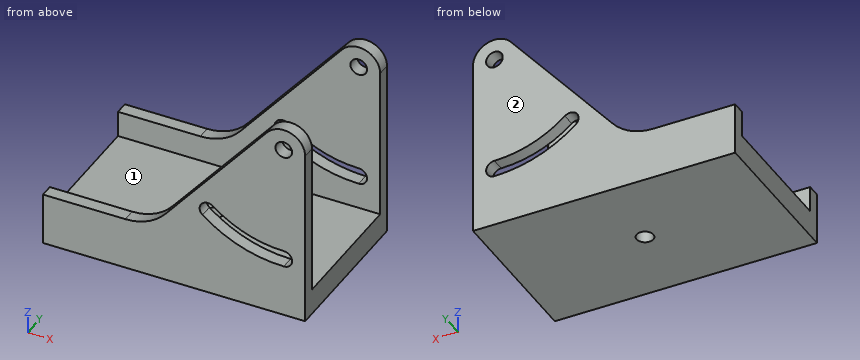
```python
from build123d import *

# Parameters (mm, degrees)
SKETCH002_W  = 100
SKETCH002_H  = 60
SKETCH002_R  = 3.175
PAD002_DEPTH = 10
SKETCH003_R  = 3.175
PAD003_DEPTH = 60
SKETCH004_W  = 50
SKETCH004_H  = 66.35
POCKET_DEPTH = 100.001


with BuildPart() as part:
    # Sketch002 → Pad002 (new body)
    with BuildSketch(Plane.XY):
        Rectangle(SKETCH002_W, SKETCH002_H)
        Circle(SKETCH002_R, mode=Mode.SUBTRACT)
    extrude(amount=PAD002_DEPTH)

    # Sketch003 (on Face1 of Pad002) → Pad003 (join)
    with BuildSketch(Plane.XZ.offset(30)):
        with BuildLine():
            ThreePointArc((50, 68.175), (44.621015, 75.856987), (35.562587, 73.429789))
            Line((-3.275594, 27.144248), (35.562587, 73.429789))
            ThreePointArc((-18.596482, 20), (-10.144117, 21.873844), (-3.275594, 27.144248))
            Line((-50, 20), (-18.596482, 20))
            Line((-50, 10), (-50, 20))
            Line((-50, 10), (50, 10))
            Line((50, 10), (50, 68.175))
        make_face()
        with Locations((41.825, 68.175)):
            Circle(SKETCH003_R, mode=Mode.SUBTRACT)
        with BuildLine():
            ThreePointArc((10.858707, 31.270809), (25.34818, 22.905308), (41.825, 20))
            ThreePointArc((41.825, 20), (45, 23.175), (41.825, 26.35))
            ThreePointArc((14.940408, 36.135191), (27.520008, 28.872356), (41.825, 26.35))
            ThreePointArc((14.940408, 36.135191), (10.467366, 35.743851), (10.858707, 31.270809))
        make_face(mode=Mode.SUBTRACT)
    extrude(amount=-PAD003_DEPTH)

    # Sketch004 (on Face15 of Pad003) → Pocket (cut, through all)
    with BuildSketch(Plane.YZ.offset(50)):
        with Locations((0, 43.175)):
            Rectangle(SKETCH004_W, SKETCH004_H)
    extrude(amount=-POCKET_DEPTH, mode=Mode.SUBTRACT)


solid = part.part
```
The model under review builds one solid part; all positions refer to its coordinate system, in mm. Face numbers are marked on the shaded views. A direction names the side the tool comes from. Give positions to 0.01 mm unless a question says otherwise; leave off trailing zeros. Write each loop counter-clockwise with the first axis right and the second up, starting at its lowest first coordinate (ties: lowest second). Pieces come first, ordered by that corner, then holes.
(1) Consider section D-D, the plane x = 0. Give the boundary of the cut face in (y, z) (3 decimals), and give its area (3 significant figures).
(2) Consider section C-C, the plane x = 17. Give the boundary of the cut face in (y, z), and give its area (3 significant figures).
(3) For P1, Ø5.5, axis at x = -39.5, y = -27.5, coming from the +Z side; P2, Ø10, axis at y = -22, z = 56.5, coming from the -X side; P3, Ø25, axis at x = 10.5, y = -7, coming from the +Z side, all flat-tipped, find the tip position at first contact; note any pin that passes through.
(4) To check wall thickness, follow L1, parallel to Y at x = 0, z = 7 (3 decimals); L2, parallel to Y at x = 8, z = 26.5; L3, parallel to Z at x = -30.5, y = 9. State the ranges of each line that lie inside material, in increasing order.
(5) Consider section B-B, the plane y = 0. Give the boundary of the cut face in (x, z) (3 decimals).
(6) Tool access review of the marked faces 1 and 2: name each direction out of +Z, -Z, +X, -X, +Y, -Y from which nothing blocks a thin tool from reaching the whole face with its end or side.
(7) Consider section A-A, the plane z = 17. Give the boundary of the cut face in (x, y).
Returned:
1. outline: (-30, 0) - (-3.175, 0) - (-3.175, 10) - (-25, 10) - (-25, 31.048) - (-30, 31.048) - close; (3.175, 0) - (30, 0) - (30, 31.048) - (25, 31.048) - (25, 10) - (3.175, 10) - close
1. area: 747 mm2
2. outline: (-30, 0) - (30, 0) - (30, 26.89) - (25, 26.89) - (25, 10) - (-25, 10) - (-25, 26.89) - (-30, 26.89) - close; (-30, 34.51) - (-25, 34.51) - (-25, 51.31) - (-30, 51.31) - close; (25, 34.51) - (30, 34.51) - (30, 51.31) - (25, 51.31) - close
2. area: 937 mm2
3. P1: stops at z = 20
3. P2: stops at x = 18
3. P3: stops at z = 10
4. L1: y = -30 to -3.175, 3.175 to 30
4. L2: y = -30 to -25, 25 to 30
4. L3: z = 0 to 10
5. outline: (-50, 0) - (-3.175, 0) - (-3.175, 10) - (-50, 10) - close; (3.175, 0) - (50, 0) - (50, 10) - (3.175, 10) - close
6. face 1: +Z, +X, -X
6. face 2: +Z, -Z, +X, -X, +Y
7. outline: (-50, -30) - (50, -30) - (50, -25) - (-50, -25) - close; (-50, 25) - (50, 25) - (50, 30) - (-50, 30) - close
